```python
from build123d import *

# Parameters (mm, degrees)
SKETCH1_W                      = 36.5
SKETCH1_H                      = 14.5
BOSS_EXTRUDE1_DEPTH            = 12
SKETCH2_W                      = 30.5
SKETCH2_H                      = 8.5
CUT_EXTRUDE1_DEPTH             = 42.067018397
F_4_5_4_5_DIAMETER_HOLE1_D     = 4.5
F_4_5_4_5_DIAMETER_HOLE1_DEPTH = 36.5
F_3_4_3_4_DIAMETER_HOLE1_D     = 3.4
F_3_4_3_4_DIAMETER_HOLE1_DEPTH = 14.5
CHAMFER1_SIZE                  = 4


with BuildPart() as part:
    # Sketch1 → Boss-Extrude1 (new body)
    with BuildSketch(Plane(origin=(7.22, 0, 0), x_dir=(0, 0, -1), z_dir=(1, 0, 0))):
        with Locations((-18.25, -7.25)):
            Rectangle(SKETCH1_W, SKETCH1_H)
    extrude(amount=-BOSS_EXTRUDE1_DEPTH)

    # Sketch2 → Cut-Extrude1 (cut, through all)
    with BuildSketch(Plane.ZY.offset(4.78)):
        with Locations((21.25, -10.25)):
            Rectangle(SKETCH2_W, SKETCH2_H)
    extrude(amount=-CUT_EXTRUDE1_DEPTH, mode=Mode.SUBTRACT)

    # Ø4.5 (4.5) Diameter Hole1
    with Locations(Plane(origin=(0, 0, 0), x_dir=(-1, 0, 0), z_dir=(0, 0, -1))):
        with Locations((-1.22, -10.25)):
            Hole(F_4_5_4_5_DIAMETER_HOLE1_D / 2, depth=F_4_5_4_5_DIAMETER_HOLE1_DEPTH)

    # Ø3.4 (3.4) Diameter Hole1
    with Locations(Plane(origin=(0, 0, 0), x_dir=(1, 0, 0), z_dir=(0, 1, 0))):
        with Locations((0, -30.98)):
            Hole(F_3_4_3_4_DIAMETER_HOLE1_D / 2, depth=F_3_4_3_4_DIAMETER_HOLE1_DEPTH)

    # Chamfer1
    chamfer1_edges = [part.edges().sort_by_distance(p)[0] for p in [
        (7.22, -14.5, 3),
    ]]
    chamfer(chamfer1_edges, length=CHAMFER1_SIZE)


solid = part.part
```
Here's how the part is built. I have some questions about the finished solid (model axes, mm). A direction names the side the tool comes from. Coordinates: 2 decimals unless noted, no trailing zeros. Write each loop counter-clockwise with the first axis right and the second up, starting at its lowest first coordinate (ties: lowest second). Pieces come first, ordered by that corner, then holes. Notation, with made-up numbers: (50.5, -39) -> (68.5, -39) arc R25 cw to (68.5, -7) -> close; hole circle Ø4 at (28.25, -35.75). An arc over 180 degrees is marked (long way). Use a Markdown table: item, result. Add a question column.
(1) For faces 4 (the flat face through (1, -7, 0)), 5 (the flat face through (0, -8, 6)), which set-ups out of +Z, -Z, +X, -X, +Y, -Y let a thin tool reach every point of the face, with its end or its side?
(2) If we section it at A-A, the plane x = 2.5: Write out the boundary of the cut face in (y, z).
(3) Please list where these lines run through material, in increasing order: line 1 (Z direction, x = 0, y = -3.2); line 2 (Y direction, x = 1.22, z = 3.9); line 3 (X direction, y = -2.5, z = 30.98).
(4) We'd pull the mould along X, two halves only. Please class faces 1 (the flat face through (-1, -14.5, 3)), 2 (the flat face through (-4.78, -4, 19)), 3 (the cylindrical face through (0.37, -3.04, 32.64)): +X half, -X half, draft (parallel to the pull), parting line (faces both ways), or undercut.
(5) If we section it at B-B, the plane z = 30.98: Write out the boundary of the cut face in (x, y), and give its area (3 significant figures).
(6) If we section it at C-C, the plane y = -5: Write out the boundary of the cut face in (x, z), and give its area (3 significant figures).
(7) I'm going to push flat-ended pins straight in: P1, Ø1.5, axis at x = -3, z = 17, coming from the +Y side; P2, Ø6, axis at x = 2.5, z = 26.5, coming from the -Y side; P3, Ø4, axis at x = 0, y = -11.5, coming from the +Z side. Where does each tip first touch, or does it pass through?
(8) If we section it at D-D, the plane x = 0: Write out the boundary of the cut face in (y, z), and give its area (3 significant figures).
Outcome:
| question | item | result |
|---|---|---|
| 1 | face 4 | -Z, +X, -X, +Y, -Y |
| 1 | face 5 | +Z, +X, -X, -Y |
| 2 | outline | (-14.5, 0) -> (-12.1, 0) -> (-12.1, 6) -> (-14.5, 6) -> close; (-8.4, 0) -> (0, 0) -> (0, 36.5) -> (-6, 36.5) -> (-6, 6) -> (-8.4, 6) -> close |
| 3 | line 1 | z = 0 to 29.28, 32.68 to 36.5 |
| 3 | line 2 | y = -14.5 to -12.5, -8 to 0 |
| 3 | line 3 | x = -4.78 to -1.7, 1.7 to 7.22 |
| 4 | face 1 | draft |
| 4 | face 2 | -X half |
| 4 | face 3 | undercut |
| 5 | outline | (-4.78, -6) -> (-1.7, -6) -> (-1.7, 0) -> (-4.78, 0) -> close; (1.7, -6) -> (7.22, -6) -> (7.22, 0) -> (1.7, 0) -> close |
| 5 | area | 51.6 mm^2 |
| 6 | outline | (-4.78, 0) -> (7.22, 0) -> (7.22, 36.5) -> (-4.78, 36.5) -> close; hole circle Ø3.4 at (0, 30.98) |
| 6 | area | 429 mm^2 |
| 7 | P1 | stops at y = 0 |
| 7 | P2 | stops at y = -6 |
| 7 | P3 | stops at z = 6 |
| 8 | outline | (-14.5, 0) -> (-12.14, 0) -> (-12.14, 6) -> (-14.5, 6) -> close; (-8.36, 0) -> (0, 0) -> (0, 29.28) -> (-6, 29.28) -> (-6, 6) -> (-8.36, 6) -> close; (-6, 32.68) -> (0, 32.68) -> (0, 36.5) -> (-6, 36.5) -> close |
| 8 | area | 227 mm^2 |
